Check sheet for the drawn part. Datum: minimum x, y, z corner. Units: mm. Give positions to 0.01 mm unless a question says otherwise; leave off trailing zeros. Order: outer loops, then holes, each group sorted by start corner. A loop starts at its lowest first (then second) coordinate and runs counter-clockwise, first axis right, second up. Notation, with made-up numbers: (-25.5, 51) - (12.5, 51) arc R30 ccw to (12.5, 86) - close; hole circle Ø1 at (60.5, 71). An arc over 180 degrees is marked (long way). Answer as a JSON object with one key per item and string values. Group by question number.
(1) Section check B-B (z = 41.5). Record the boundary of the cut face in (x, y) (1 decimal).
(2) Section check C-C (z = 61.5). Record the boundary of the cut face in (x, y) (1 decimal).
(3) Thickness scan on line 1 (X direction, y = 1.15, z = 29); line 2 (X direction, y = 1.3, z = 33) (1 decimal). Record the ranges inside material, lowest first.
(4) Section check A-A (y = 0.6). Record the boundary of the cut face in (x, z).
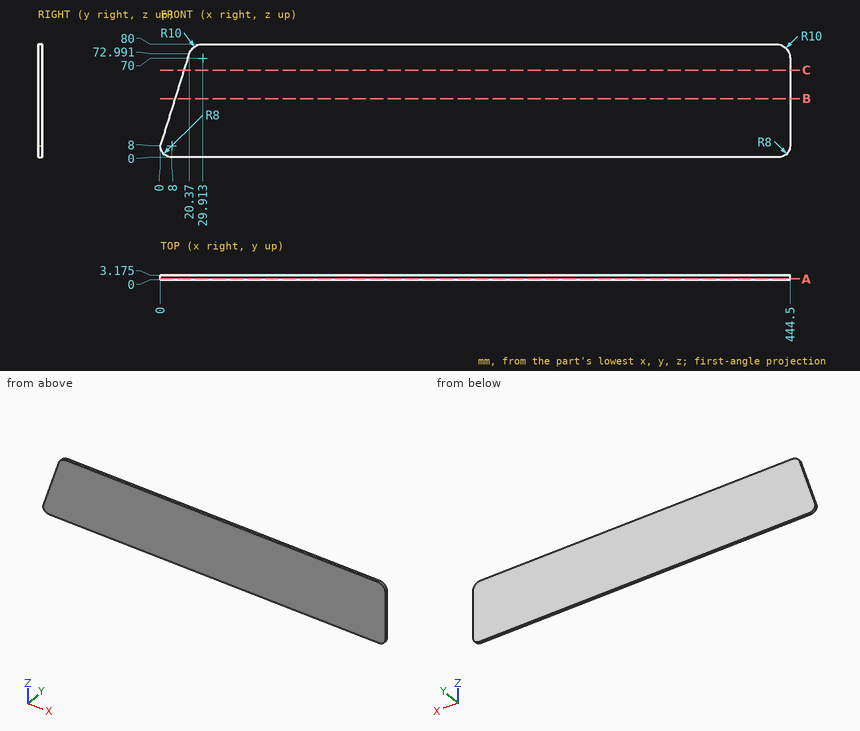
Solutions:
{
 "1": {"outline": "(10.5, 0) - (444.5, 0) - (444.5, 3.2) - (10.5, 3.2) - close"},
 "2": {"outline": "(16.8, 0) - (444.5, 0) - (444.5, 3.2) - (16.8, 3.2) - close"},
 "3": {"line 1": "x = 6.58 to 444.5", "line 2": "x = 7.8 to 444.5"},
 "4": {"outline": "(0, 8) arc R8 ccw to (8, 0) - (436.5, 0) arc R8 ccw to (444.5, 8) - (444.5, 70) arc R10 ccw to (434.5, 80) - (29.91, 80) arc R10 ccw to (20.37, 72.99) - close"}
}
